Read the model definition and answer for the solid it produces. Units are mm, in the model's axes. Face numbers are marked on the shaded views. A direction names the side the tool comes from. Round coordinates to 2 decimals unless told otherwise and drop trailing zeros. Loops run counter-clockwise (first coordinate to the right, second up) from the corner with the lowest first, then second, coordinate; pieces in that order, holes last. Notation, with made-up numbers: M 20,17 L 38,17 A17 cw 38,22 Z; hole C 80.5,9 d5. An arc over 180 degrees is marked long. Write each question's results on one line, items separated by ' | '.
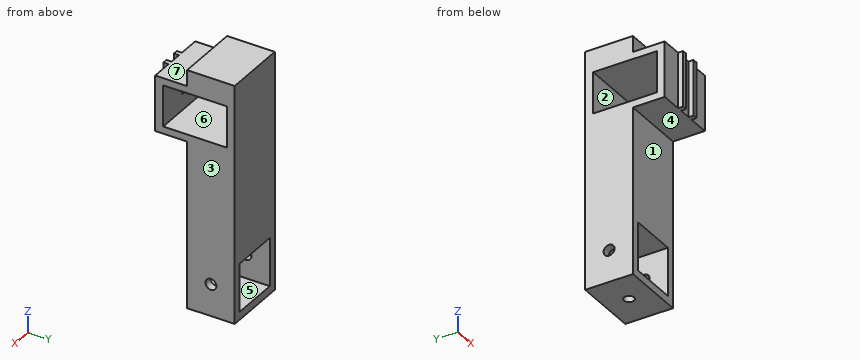
Autodesk Inventor part; units mm, degrees
ref_plane "YZ Plane" through (0, 0, 0) normal (1, 0, 0) x (0, 1, 0)
ref_plane "XZ Plane" through (0, 0, 0) normal (0, 1, 0) x (-1, 0, 0)
ref_plane "XY Plane" through (0, 0, 0) normal (0, 0, 1) x (1, 0, 0)
sketch "스케치1" plane through (0, 0, 0) normal (0, 1, 0) x (-1, 0, 0)
  line L0 (40.4, 0) -> (0, 0)
  line L1 (0, 0) -> (0, -150)
  line L2 (0, -150) -> (40.4, -150)
  line L3 (40.4, -150) -> (40.4, 0)
  line L4 (35.4, -114.6) -> (5, -114.6)
  line L5 (5, -114.6) -> (5, -145)
  line L6 (5, -145) -> (35.4, -145)
  line L7 (35.4, -145) -> (35.4, -114.6)
  line L8 (20.2, -114.6) -> (20.2, -145) construction
  line L9 (35.4, -129.8) -> (5, -129.8) construction
  line L10 (35.65, -10) -> (4.75, -10)
  line L11 (4.75, -10) -> (4.75, -80)
  line L12 (4.75, -80) -> (35.65, -80)
  line L13 (35.65, -80) -> (35.65, -10)
  point P0 (20.2, -150)
  dimension "d0" = 30.4
  dimension "d1" = 30.4
  dimension "d2" = 5
  dimension "d3" = 5
  dimension "d4" = 5
  dimension "d5" = 70
  dimension "d6" = 4.75
  dimension "d7" = 4.75
  dimension "d8" = 10
  dimension "d9" = 150
extrude "돌출1" add sketch "스케치1" along normal blind 30
sketch "스케치2" plane through (0, 0, 0) normal (1, 0, 0) x (0, 0, -1)
  circle A0 centre (130, 15) radius 3.45
  line L0 (150, 0) -> (150, 30)
  line L1 (0, 30) -> (150, 30)
  point P0 (0, 0)
  dimension "d12" = 20
  dimension "d13" = 15
  dimension "d14" = 6.9
extrude "돌출2" cut sketch "스케치2" against normal blind 50
sketch "스케치3" plane through (0, 0, -150) normal (0, 0, -1) x (-1, 0, 0)
  circle A0 centre (20.2, 15) radius 3.15
  line L0 (0, 30) -> (40.4, 30)
  line L1 (40.4, 0) -> (40.4, 30)
  point P0 (0, 0)
  point P1 (20.2, 30)
  point P2 (40.4, 15)
  dimension "d17" = 6.3
extrude "돌출3" cut sketch "스케치3" against normal blind 10
extrude "돌출5" add sketch "스케치1" along normal up to surface (30 mm away) contours L13 L12 L11 L10
sketch "스케치5" plane through (0, 0, 0) normal (0, -1, 0) x (1, 0, 0)
  line L0 (-4.75, -10) -> (-35.65, -10)
  line L1 (-35.65, -10) -> (-35.65, -45)
  line L2 (-35.65, -45) -> (-4.75, -45)
  line L3 (-4.75, -45) -> (-4.75, -10)
  line L4 (-4.75, -10) -> (-4.75, -80)
  line L5 (-35.65, -10) -> (-4.75, -10)
  line L6 (0, -10) -> (-40.4, -10)
  line L7 (-40.4, -10) -> (-40.4, -45)
  line L8 (-40.4, -45) -> (0, -45)
  line L9 (0, -45) -> (0, -10)
  line L10 (0, 0) -> (0, -150)
  line L11 (-40.4, -150) -> (-40.4, 0)
  line L12 (-40.4, -150) -> (-40.4, 0)
  point P0 (-4.75, -45)
  dimension "d27" = 35
extrude "돌출6" add sketch "스케치5" along normal blind 20
sketch "스케치6" plane through (0, 0, -150) normal (1, 0, 0) x (0, 0, -1)
  line L0 (-135.5, -15) -> (-109.5, -15)
  line L1 (-109.5, -15) -> (-109.5, 25)
  line L2 (-109.5, 25) -> (-135.5, 25)
  line L3 (-135.5, 25) -> (-135.5, -15)
  line L4 (-150, 30) -> (0, 30)
  line L5 (-105, -20) -> (-140, -20)
  line L6 (-140, 0) -> (-140, -20)
  point P0 (-150, 0)
  dimension "d30" = 5
  dimension "d31" = 5
  dimension "d32" = 26
  dimension "d33" = 4.5
extrude "돌출7" cut sketch "스케치6" against normal up to surface (40.4 mm away)
sketch "스케치7" plane through (0, -15, -14.5) normal (0, 1, 0) x (1, 0, 0)
  circle A0 centre (-20.2, 14.5) radius 1.45
  line L0 (0, -4.5) -> (-40.4, -4.5)
  line L1 (-40.4, 30.5) -> (0, 30.5)
  point P0 (0, -14.5)
  point P1 (-20.2, 30.5)
  dimension "d36" = 2.9
  dimension "d37" = 19
extrude "돌출8" cut sketch "스케치7" against normal blind 10
sketch "스케치8" plane through (0, -20, 0) normal (0, -1, 0) x (1, 0, 0)
  line L0 (0, -10) -> (-40.4, -10)
  line L1 (-13.4, -10) -> (-16.4, -10)
  line L2 (-16.4, -10) -> (-16.4, -45)
  line L3 (-16.4, -45) -> (-13.4, -45)
  line L4 (-13.4, -45) -> (-13.4, -10)
  line L5 (-24, -10) -> (-27, -10)
  line L6 (-27, -10) -> (-27, -45)
  line L7 (-27, -45) -> (-24, -45)
  line L8 (-24, -45) -> (-24, -10)
  line L9 (-40.4, -45) -> (0, -45)
  circle A0 centre (-20.2, -29) radius 1.45
  point P0 (0, 0)
  dimension "d40" = 7.6
  dimension "d41" = 3.8
  dimension "d42" = 3
  dimension "d43" = 3
extrude "돌출9" add sketch "스케치8" along normal blind 3.2 contours L4 L3 L2 L0 | L8 L7 L6 L0
properties part number "lever_support"
1. Find section B-B, the plane y = 15. Give the vertices of the cut face in (x, z).
Completed:
outline: M -40.4,-150 L -23.35,-150 L -23.35,-145 L -35.4,-145 L -35.4,-133.45 L -40.4,-133.45 Z; M -40.4,-126.55 L -35.4,-126.55 L -35.4,-114.6 L -5,-114.6 L -5,-126.55 L 0,-126.55 L 0,-40.5 L -40.4,-40.5 Z; M -40.4,-14.5 L 0,-14.5 L 0,0 L -40.4,0 Z; M -17.05,-150 L 0,-150 L 0,-133.45 L -5,-133.45 L -5,-145 L -17.05,-145 Z
2. Given P1, Ø1.6, axis at y = -21, z = -24.5, coming from the -X side; P2, Ø7, axis at x = -20.2, y = 15, coming from the -Z side; P3, Ø2, axis at x = -23, y = -14, coming from the +Z side; P4, Ø1, axis at y = -22, z = -24, coming from the +X side, each flat-ended and moving along its own axis, determine where each tip first touches the part or whether it passes through.
Completed:
P1: stops at x = -27 | P2: stops at z = -150 | P3: stops at z = -10 | P4: stops at x = -13.4
3. Find section A-A, the plane x = -20.2. Give the vertices of the cut face in (y, z), then the cut area to 3 significant figures.
Completed:
outline: M -20,-45 L 0,-45 L 0,-114.6 L 30,-114.6 L 30,0 L 0,0 L 0,-10 L -20,-10 L -20,-27.55 L -15,-27.55 L -15,-14.5 L 25,-14.5 L 25,-40.5 L -15,-40.5 L -15,-30.45 L -20,-30.45 Z; M 0,-150 L 11.85,-150 L 11.85,-145 L 0,-145 Z; M 18.15,-150 L 30,-150 L 30,-145 L 18.15,-145 Z | area: 3,200 mm2
4. Find the intervals of material crossed by L1, parallel to Z at x = -6.5, y = 20; L2, parallel to Y at x = -37.2, z = -130; L3, parallel to X at y = -18, z = -29, in increasing order.
Completed:
L1: z = -150 to -145, -114.6 to -40.5, -14.5 to 0 | L2: y = 0 to 11.55, 18.45 to 30 | L3: x = -40.4 to -21.65, -18.75 to 0
5. Which of the six approach directions +Z, -Z, +X, -X, +Y, -Y give full straight-line access (tool end or side, diameter ignored) to the marked faces 4, 5, 6 and 7?
Completed:
face 4: -Z, +X, -X, -Y | face 5: +Y, -Y | face 6: +X, -X | face 7: +Z, +X, -X, -Y
6. Find section C-C, the plane z = -29. Give the vertices of the cut face in (x, y), then the cut area to 3 significant figures.
Completed:
outline: M -40.4,-20 L -27,-20 L -27,-23.2 L -24,-23.2 L -24,-20 L -21.65,-20 L -21.65,-15 L -40.4,-15 Z; M -40.4,25 L 0,25 L 0,30 L -40.4,30 Z; M -18.75,-20 L -16.4,-20 L -16.4,-23.2 L -13.4,-23.2 L -13.4,-20 L 0,-20 L 0,-15 L -18.75,-15 Z | area: 409 mm2
7. Determine the mould class of the marked faces 1, 2 and 3 for opening direction Y: released by +Y, released by -Y, zero draft, split by the parting line, or undercut.
Completed:
face 1: released by -Y | face 2: undercut | face 3: zero draft
8. Find section D-D, the plane y = 7. Give the vertices of the cut face in (x, z), then the cut area to 3 significant figures.
Completed:
outline: M -40.4,-150 L 0,-150 L 0,-40.5 L -40.4,-40.5 Z; M -40.4,-14.5 L 0,-14.5 L 0,0 L -40.4,0 Z; hole M -35.4,-145 L -5,-145 L -5,-114.6 L -35.4,-114.6 Z | area: 4,090 mm2
